Autodesk Inventor part; units mm, degrees
ref_plane "YZ Plane" through (0, 0, 0) normal (1, 0, 0) x (0, 1, 0)
ref_plane "XZ Plane" through (0, 0, 0) normal (0, 1, 0) x (-1, 0, 0)
ref_plane "XY Plane" through (0, 0, 0) normal (0, 0, 1) x (1, 0, 0)
sketch "Sketch1" plane through (0, 0, 0) normal (0, 1, 0) x (-1, 0, 0)
  circle A0 centre (0, 0) radius 5
  dimension "d0" = 10
extrude "Extrusion1" add sketch "Sketch1" along normal blind 17
sketch "Sketch2" plane through (0, 17, 0) normal (0, 1, 0) x (1, 0, 0)
  line L0 (0, 0) -> (-2, 0)
  line L1 (-2, 0) -> (-2, 7.2521)
  line L2 (0, 0) -> (2, 0)
  line L3 (2, 0) -> (2, -7.0492)
  line L4 (2, -7.0492) -> (-2, -7.0492)
  line L5 (-2, -7.0492) -> (-2, 7.2521)
  line L6 (-2, 7.2521) -> (2, 7.2521)
  line L7 (2, 7.2521) -> (2, -7.0492)
  line L8 (-2, -7.0492) -> (-8.2773, -7.0492)
  line L9 (-8.2773, -7.0492) -> (-8.2773, 7.6578)
  line L10 (-8.2773, 7.6578) -> (-2, 7.6578)
  line L11 (-2, 7.6578) -> (-2, -7.0492)
  line L12 (2, 7.2521) -> (6.5688, 7.2521)
  line L13 (6.5688, 7.2521) -> (6.5688, -6.4823)
  line L14 (6.5688, -6.4823) -> (2, -6.4823)
  line L15 (2, -6.4823) -> (2, 7.2521)
  dimension "d3" = 2
  dimension "d4" = 2
extrude "Extrusion2" cut sketch "Sketch2" against normal blind 3.5 contours L5 L8 L9 L10 L11 L1 | L7 L12 L13 L14 L3
sketch "Sketch3" plane through (2, 17, 4.5826) normal (1, 0, 0) x (0, 0, -1)
  line L0 (9.1652, 0) -> (0, 0)
  line L1 (4.5826, 0) -> (4.5826, -1.75)
  line L2 (4.5826, -1.75) -> (2.5826, -1.75)
  line L3 (4.5826, -1.75) -> (6.5826, -1.75)
  circle A0 centre (2.5826, -1.75) radius 1.1
  circle A1 centre (6.5826, -1.75) radius 1.1
  point P0 (4.5826, -17)
  dimension "d7" = 1.75
  dimension "d8" = 2
  dimension "d9" = 2
  dimension "d10" = 2.2
  dimension "d11" = 2.2
extrude "Extrusion3" cut sketch "Sketch3" against normal blind 56
properties part number "drive_shaft_v4"
Build history of the part. All positions in model axes, mm. A direction names the side the tool comes from. Round coordinates to 2 decimals unless told otherwise and drop trailing zeros. Write each loop counter-clockwise with the first axis right and the second up, starting at its lowest first coordinate (ties: lowest second). Pieces come first, ordered by that corner, then holes. Notation, with made-up numbers: M -32.75,17 L -11.75,17 A14 cw -11.75,26 Z; hole C 44,1.25 d10. An arc over 180 degrees is marked long. Answer in a Markdown table with one row per item.
1. Flat gauge pins, fed straight in: P1, Ø1, axis at y = 9.5, z = 1, coming from the -X side; P2, Ø2, axis at y = 15.25, z = 2, coming from the -X side; P3, Ø1.8, axis at y = 15, z = 0, coming from the -X side; P4, Ø1.5, axis at x = -3.5, z = -2, coming from the +Y side. Where does each tip first touch, or does it go through?
Geometry check:
| item | result |
|---|---|
| P1 | x = -4.97 |
| P2 | through |
| P3 | x = -2 |
| P4 | y = 13.5 |
2. Saw through at D-D (x = -3). List the corners of the cut face in (y, z), and give its area (3 significant figures).
Geometry check:
| item | result |
|---|---|
| outline | M 0,-4 L 13.5,-4 L 13.5,4 L 0,4 Z |
| area | 108 mm2 |
3. Saw through at C-C (x = 0). List the corners of the cut face in (y, z).
Geometry check:
| item | result |
|---|---|
| outline | M 0,-5 L 17,-5 L 17,5 L 0,5 Z; hole C 15.25,-2 d2.2; hole C 15.25,2 d2.2 |
4. Probe L1, parallel to Y at x = 0.05, z = 2; L2, parallel to Y at x = -3, z = 3.5; L3, parallel to Z at x = 2, y = 12. List the from-to ranges inside material, lowest first. Write a range as [from, to].
Geometry check:
| item | result |
|---|---|
| L1 | [0, 14.15], [16.35, 17] |
| L2 | [0, 13.5] |
| L3 | [-4.58, 4.58] |
5. Saw through at B-B (z = 0). List the corners of the cut face in (x, y), and give its area (3 significant figures).
Geometry check:
| item | result |
|---|---|
| outline | M -5,0 L 5,0 L 5,13.5 L 2,13.5 L 2,17 L -2,17 L -2,13.5 L -5,13.5 Z |
| area | 149 mm2 |
6. Which spindle directions (+Z, -Z, +X, -X, +Y, -Y) get a long thin tool onto all of the face, cutting with end or side? Do faces 1 (the face through (-2, 15, 0)), 2 (the face through (0.028, 14.176, 2.238)), 3 (the face through (2, 15, 0)). Say none if no direction does.
Geometry check:
| item | result |
|---|---|
| face 1 | +Z, -Z, -X, +Y |
| face 2 | +X, -X |
| face 3 | +Z, -Z, +X, +Y |
7. Saw through at A-A (z = 2). List the corners of the cut face in (x, y).
Geometry check:
| item | result |
|---|---|
| outline | M -4.58,0 L 4.58,0 L 4.58,13.5 L 2,13.5 L 2,14.15 L -2,14.15 L -2,13.5 L -4.58,13.5 Z; M -2,16.35 L 2,16.35 L 2,17 L -2,17 Z |
